Read the model definition and answer for the solid it produces. Units are mm, in the model's axes. Coordinates: 2 decimals unless noted, no trailing zeros. Write each loop counter-clockwise with the first axis right and the second up, starting at its lowest first coordinate (ties: lowest second). Pieces come first, ordered by that corner, then holes. Notation, with made-up numbers: M 84.25,8.5 L 111.25,8.5 A14 ccw 111.25,23.5 Z; hole C 66.25,-15 d10. An arc over 180 degrees is marked long. Write item = value, one per line.
Solid Edge part; units mm, degrees
sketch "Sketch1" plane through (0, 0, 0) normal (0, 0, 1) x (1, 0, 0)
  circle A0 centre (0, 0) radius 40
extrude "Protrusion1" add sketch "Sketch1" along normal blind 2
sketch "Sketch2" plane through (0, 0, 2) normal (0, 0, 1) x (1, 0, 0)
  circle A0 centre (0, 30) radius 4
extrude "Cutout1" cut sketch "Sketch2" against normal up to next
pattern_circular "Pattern1" count 4 over 360 about axis through (0, 0, 2) along (0, 0, 1) of "Cutout1"
Item 1: For a pull along X with two mould halves and no side action, classify faces 1 (the face through (-8.67, 39.05, 0.99)), 2 (the face through (33.966, 0.521, 1.014)), 3 (the face through (-1, 1, 0)) as released by +X, released by -X, zero draft, split by the parting line, or undercut.
Worked answers:
face_1 = split by the parting line
face_2 = undercut
face_3 = zero draft
Item 2: Find section C-C (z = 1.55). Determine the outline of the cut face in (x, y), and give its area (3 significant figures).
Worked answers:
outline = C 0,0 d80; hole C -30,0 d8; hole C 0,-30 d8; hole C 0,30 d8; hole C 30,0 d8
area = 4,830 mm²
Item 3: Find section A-A (x = 0). Determine the outline of the cut face in (y, z).
Worked answers:
outline = M -40,0 L -34,0 L -34,2 L -40,2 Z; M -26,0 L 26,0 L 26,2 L -26,2 Z; M 34,0 L 40,0 L 40,2 L 34,2 Z
Item 4: Flat-ended cylindrical pins translate along their axes: pin 1 (2 mm diameter, centred on x = -18.5, y = 10.5, fed in from -Z); pin 2 (1 mm diameter, centred on x = -1.5, z = 1, fed in from +Y). Find the tip coordinate at first contact, or state that the pin passes through.
Worked answers:
pin_1 = 0
pin_2 = 39.99
Item 5: Consider line 1 along X through (y, z) = (1.5, 0.5); line 2 along Y through (x, z) = (0.5, 1.5); line 3 along Y through (x, z) = (-28.5, 1). Determine where each line is inside the solid, lowest interval first. Write a range as from..to.
Worked answers:
line_1 = -39.97..-33.71, -26.29..26.29, 33.71..39.97
line_2 = -40..-33.97, -26.03..26.03, 33.97..40
line_3 = -28.07..-3.71, 3.71..28.07
Item 6: Find section D-D (x = -30). Determine the outline of the cut face in (y, z), and give its area (3 significant figures).
Worked answers:
outline = M -26.46,0 L -4,0 L -4,2 L -26.46,2 Z; M 4,0 L 26.46,0 L 26.46,2 L 4,2 Z
area = 89.8 mm²
